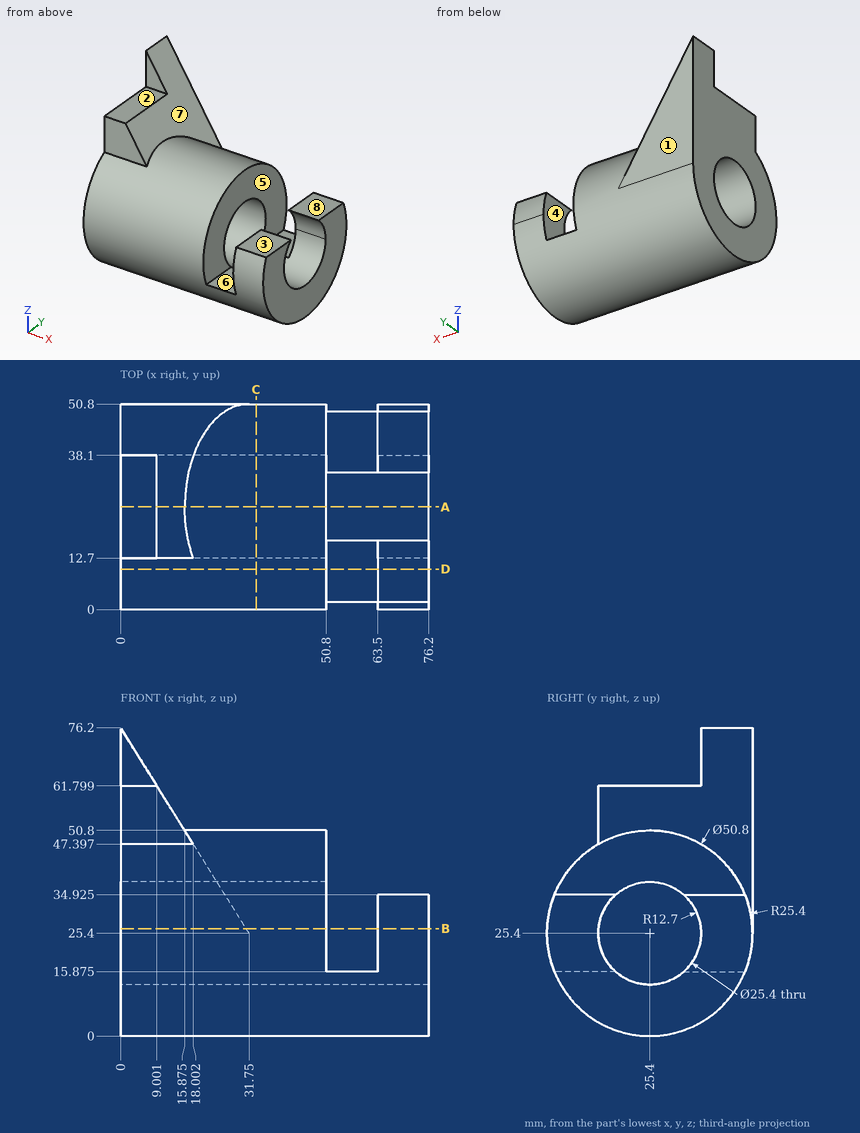
Check sheet for the drawn part. Datum: minimum x, y, z corner. Units: mm. A direction names the side the tool comes from. Round coordinates to 2 decimals unless told otherwise and drop trailing zeros. Order: outer loops, then holes, each group sorted by start corner. A loop starts at its lowest first (then second) coordinate and runs counter-clockwise, first axis right, second up. Notation, with made-up numbers: (-25.5, -15) -> (20.5, -15) arc R24 cw to (20.5, 4) -> close; hole circle Ø7 at (72.5, 44). An arc over 180 degrees is marked (long way). Return JSON: item names as keys, results as strings. Group by question number.
Q1. Section check D-D, the plane y = 10. Record the boundary of the cut face in (x, z) (1 decimal).
Q2. Section check A-A, the plane y = 25.4. Record the boundary of the cut face in (x, z) (1 decimal).
Q3. Section check B-B, the plane z = 26.5. Count the separate pieces of the cut face and the enclosed holes in it, plus the area to 3 significant figures.
Q4. Section check C-C, the plane x = 33.5. Record the boundary of the cut face in (y, z).
Q5. Release check for a two-part mould opening along X. For the marked faces 5, 6, 7 and 8 record: released by +X, released by -X, zero draft, split by the parting line, or undercut.
Q6. Gauge pin test, flat ends, axial feed: pin 1 (14 mm diameter, centred on x = 66.5, y = 42, fed in from +Z) (3 decimals); pin 2 (2.5 mm diameter, centred on x = 6, y = 29, fed in from +Z); pin 3 (10 mm diameter, centred on x = 3.5, z = 69.5, fed in from -Y). Record the tip position at first contact, or that the pin passes through.
Q7. Tool access check on the marked faces 1, 2, 3 and 4. Record the directions out of +Z, -Z, +X, -X, +Y, -Y that give a thin tool (end or side, any length) a straight path to the whole face; none if there is none.
Q8. Material ranges on probe 1 along Z at (x, y) = (26, 25); probe 2 along Z at (x, y) = (54, 25); probe 3 along Y at (x, z) = (8, 48.5), recorded low to high. Write a range as from..to.
Numbers:
{
 "1": {"outline": "(0, 5.2) -> (76.2, 5.2) -> (76.2, 34.9) -> (63.5, 34.9) -> (63.5, 15.9) -> (50.8, 15.9) -> (50.8, 45.6) -> (0, 45.6) -> close"},
 "2": {"outline": "(0, 0) -> (76.2, 0) -> (76.2, 12.7) -> (0, 12.7) -> close; (0, 38.1) -> (50.8, 38.1) -> (50.8, 50.8) -> (15.9, 50.8) -> (9, 61.8) -> (0, 61.8) -> close"},
 "3": {"separate pieces": "4", "enclosed holes": "0", "area": "1,620 mm^2"},
 "4": {"outline": "circle Ø50.8 at (25.4, 25.4); hole circle Ø25.4 at (25.4, 25.4)"},
 "5": {"face 5": "undercut", "face 6": "undercut", "face 7": "released by +X", "face 8": "zero draft"},
 "6": {"pin 1": "z = 34.925", "pin 2": "z = 61.8", "pin 3": "y = 38.1"},
 "7": {"face 1": "+Z, -Z, +X, -X, +Y", "face 2": "+Z, +X, -X, -Y", "face 3": "+Z, +X, +Y, -Y", "face 4": "+Z, +Y, -Y"},
 "8": {"probe 1": "0..12.71, 38.09..50.8", "probe 2": "0..12.71", "probe 3": "12.7..50.8"}
}
